from build123d import *

# Parameters (mm, degrees)
F0_W     = 76.2
F0_H     = 50.8
F1_DEPTH = 12.7
F3_DEPTH = 5.08
F4_R     = 1.5875
F5_DEPTH = 25.4
F6_R     = 4.7625
F7_DEPTH = 0.889


with BuildPart() as f1:
    # F0 (on Top) → F1 (new body)
    with BuildSketch(Plane.XY):
        with Locations((1.773075, -0.713211)):
            Rectangle(F0_W, F0_H)
    extrude(amount=F1_DEPTH)

    # F2 (on face) → F3 (cut)
    with BuildSketch(Plane.XY.offset(12.7)):
        with BuildLine():
            Line((-2.955125, 9.086431), (-2.955125, 24.686789))
            Line((-2.955125, 24.686789), (-36.326925, 24.686789))
            Line((-36.326925, 24.686789), (-36.326925, -26.113211))
            Line((-36.326925, -26.113211), (24.675291, -26.113211))
            Line((24.675291, -26.113211), (24.675291, 5.911431))
            ThreePointArc((24.675291, 5.911431), (26.920355, 11.331495), (21.500291, 9.086431))
            Line((21.500291, 9.086431), (-2.955125, 9.086431))
        make_face()
    extrude(amount=-F3_DEPTH, mode=Mode.SUBTRACT)

    # F4 (on face) → F5 (cut)
    with BuildSketch(Plane.XY.offset(7.62)):
        with Locations((6.704791, -3.472849)):
            Circle(F4_R)
    extrude(amount=-F5_DEPTH, mode=Mode.SUBTRACT)

    # F6 (on face) → F7 (cut)
    with BuildSketch(Plane.XY.offset(7.62)):
        with Locations((6.704791, -3.472849)):
            Circle(F6_R)
    extrude(amount=-F7_DEPTH, mode=Mode.SUBTRACT)


solid = f1.part
Geometry: final body of the model. Coordinates: model frame, mm. A direction names the side the tool comes from. Coordinates: 2 decimals unless noted, no trailing zeros. Loops run counter-clockwise (first coordinate to the right, second up) from the corner with the lowest first, then second, coordinate; pieces in that order, holes last. Notation, with made-up numbers: (-26.5, -8.75) - (17.5, -8.75) arc R28 cw to (17.5, 17.25) - close; hole circle Ø3 at (3.5, 41.5). An arc over 180 degrees is marked (long way). Put each result on its own line as item: value. Start each with the question number.
Q1. Cut plane D-D, the plane x = -9.5. Return loops of the section in (y, z).
Q2. Pin query (flat end, axial travel): pin 1 Ø5 at (x, y) = (9, -5.5) entering from +Z; pin 2 Ø2.5 at (y, z) = (20, 9.5) entering from -X; pin 3 Ø1.5 at (x, z) = (8.5, 10) entering from -Y. Return the tip coordinate at first contact, or that it passes through.
Q3. Cut plane C-C, the plane y = 14.5. Return loops of the section in (x, z).
Q4. Pull-direction query (Y, two-part tool) for faces 1 (the flat face through (10, -26.113, 5)), 2 (the flat face through (39.873, -1, 6)), 3 (the cylindrical face through (11.104, -5.297, 7.182)); classes: released by +Y, released by -Y, zero draft, split by the parting line, or undercut.
Q5. Set-up query: faces 4 (the flat face through (-36.327, -1, 4)), 5 (the flat face through (-2.955, 17, 10)), 6 (the flat face through (7, -6, 6.731)), 7 (the flat face through (28, 5, 12.7)), 8 (the flat face through (9, 9.086, 10)). Return all of +Z, -Z, +X, -X, +Y, -Y with unobstructed straight access to the full face (end or side cutting, diameter ignored); none if empty.
Q6. Cut plane B-B, the plane x = 1. Return loops of the section in (y, z), and give its area (3 significant figures).
Q7. Line query: line 1 (Z direction, x = 0, y = 5.5); line 2 (Y direction, x = 27, z = 11.5); line 3 (X direction, y = -11.5, z = 11.25). Output: solid intervals per line, ascending.
Q8. Cut plane A-A, the plane z = 8.5. Return loops of the section in (x, y) (3 decimals).
Filled sheet:
1. outline: (-26.11, 0) - (24.69, 0) - (24.69, 7.62) - (-26.11, 7.62) - close
2. pin 1: z = 7.62
2. pin 2: x = -2.96
2. pin 3: y = 9.09
3. outline: (-36.33, 0) - (39.87, 0) - (39.87, 12.7) - (-2.96, 12.7) - (-2.96, 7.62) - (-36.33, 7.62) - close
4. face 1: released by -Y
4. face 2: zero draft
4. face 3: undercut
5. face 4: +Z, -Z, -X, +Y, -Y
5. face 5: +Z, -X, +Y, -Y
5. face 6: +Z
5. face 7: +Z, +X, -X, +Y, -Y
5. face 8: +Z, -X, -Y
6. outline: (-26.11, 0) - (24.69, 0) - (24.69, 12.7) - (9.09, 12.7) - (9.09, 7.62) - (-26.11, 7.62) - close
6. area: 466 mm²
7. line 1: 0 to 7.62
7. line 2: -26.11 to 6.92, 11.25 to 24.69
7. line 3: 24.68 to 39.87
8. outline: (-2.955, 9.086) - (21.5, 9.086) arc R3.175 cw (long way) to (24.675, 5.911) - (24.675, -26.113) - (39.873, -26.113) - (39.873, 24.687) - (-2.955, 24.687) - close
